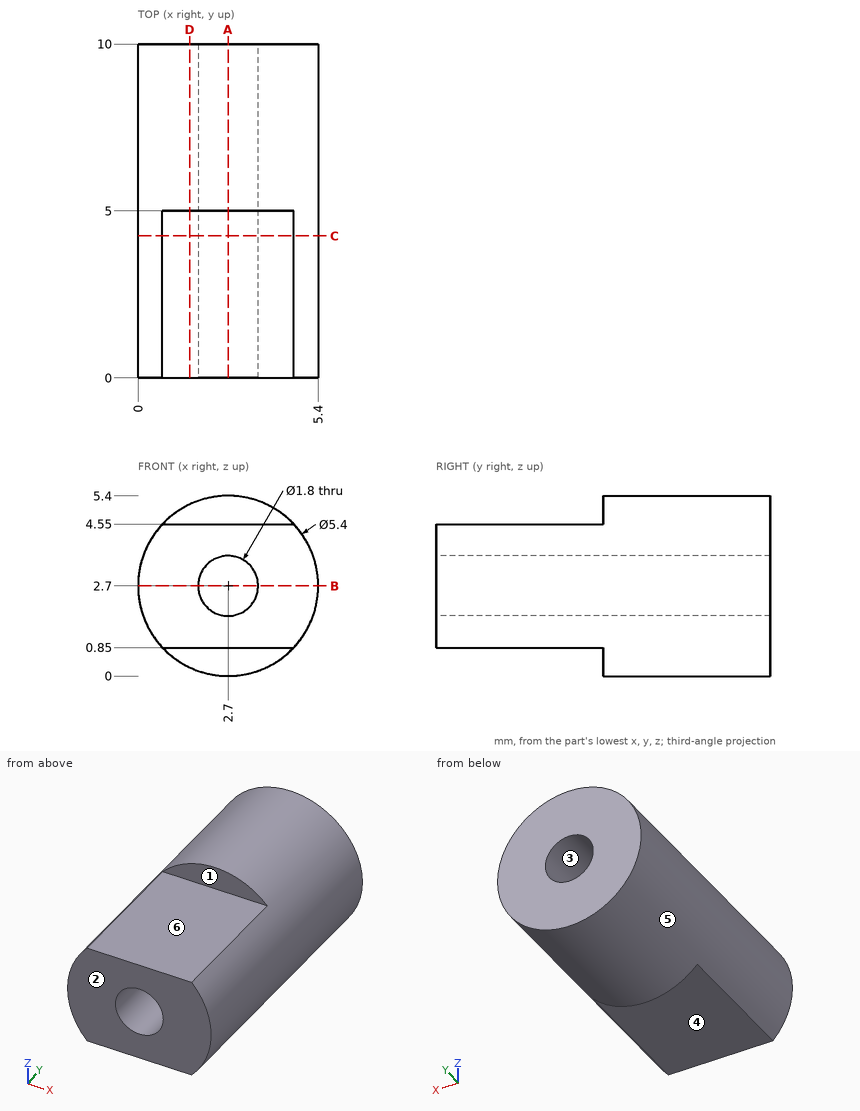
Part print with two shaded views. Sizes in mm from the minimum x, y, z corner. A direction names the side the tool comes from. Coordinates: 2 decimals unless noted, no trailing zeros. Write each loop counter-clockwise with the first axis right and the second up, starting at its lowest first coordinate (ties: lowest second). Pieces come first, ordered by that corner, then holes. Notation, with made-up numbers: (-19.5, 14.5) - (14.5, 14.5) arc R29 ccw to (14.5, 45.5) - close; hole circle Ø8 at (85.25, -13). An arc over 180 degrees is marked (long way). Use a Markdown table: item, result. Add a question column.
Item 1: 3-axis set-ups, long thin cutter, end or side, ignore diameter. For the marked faces 1 and 2: which of +Z, -Z, +X, -X, +Y, -Y reach the whole face in a straight line?
Item 2: Band-saw the part on B-B, the plane z = 2.7. Write the cut outline in (x, y), and give its area (3 significant figures).
Item 3: Band-saw the part on D-D, the plane x = 1.55. Write the cut outline in (y, z), and give its area (3 significant figures).
Item 4: Band-saw the part on A-A, the plane x = 2.7. Write the cut outline in (y, z).
Item 5: Drop flat-ended pins along their axis: pin 1 (3 mm diameter, centred on x = 3, y = 3, fed in from -Z); pin 2 (3 mm diameter, centred on x = 0.5, z = 4.5, fed in from +Y); pin 3 (0.7 mm diameter, centred on x = 2.5, z = 5, fed in from -Y); pin 4 (2 mm diameter, centred on x = 3.5, y = 3, fed in from +Z). Give the stop position or say it passes through.
Item 6: Two-plate mould, pull along Z, no slides. Class the marked faces 3, 4, 5 and 6: pulls with the +Z half, pulls with the -Z half, needs draft (parallel to the pull), parting line crosses it, or undercut.
Item 7: Drill centre lines: line 1 along Z through (x, y) = (2.7, 6.5); line 2 along Z through (x, y) = (2.7, 4). Where is each one in solid material? Low to high.
Item 8: Band-saw the part on C-C, the plane y = 4.25. Write the cut outline in (x, z).
A:
| question | item | result |
|---|---|---|
| 1 | face 1 | +Z, +X, -X, -Y |
| 1 | face 2 | +Z, -Z, +X, -X, -Y |
| 2 | outline | (0, 0) - (1.8, 0) - (1.8, 10) - (0, 10) - close; (3.6, 0) - (5.4, 0) - (5.4, 10) - (3.6, 10) - close |
| 2 | area | 36.0 mm² |
| 3 | outline | (0, 0.85) - (5, 0.85) - (5, 0.26) - (10, 0.26) - (10, 5.14) - (5, 5.14) - (5, 4.55) - (0, 4.55) - close |
| 3 | area | 42.9 mm² |
| 4 | outline | (0, 0.85) - (5, 0.85) - (5, 0) - (10, 0) - (10, 1.8) - (0, 1.8) - close; (0, 3.6) - (10, 3.6) - (10, 5.4) - (5, 5.4) - (5, 4.55) - (0, 4.55) - close |
| 5 | pin 1 | stops at z = 0.85 |
| 5 | pin 2 | stops at y = 10 |
| 5 | pin 3 | stops at y = 5 |
| 5 | pin 4 | stops at z = 4.55 |
| 6 | face 3 | undercut |
| 6 | face 4 | pulls with the -Z half |
| 6 | face 5 | parting line crosses it |
| 6 | face 6 | pulls with the +Z half |
| 7 | line 1 | z = 0 to 1.8, 3.6 to 5.4 |
| 7 | line 2 | z = 0.85 to 1.8, 3.6 to 4.55 |
| 8 | outline | (0.73, 0.85) - (4.67, 0.85) arc R2.7 ccw to (4.67, 4.55) - (0.73, 4.55) arc R2.7 ccw to start; hole circle Ø1.8 at (2.7, 2.7) |
